from build123d import *

# Parameters (mm, degrees)
BOSS_EXTRUDE1_DEPTH        = 10
M4_TAPPED_HOLE1_AT_2_COUNT = 2
M4_TAPPED_HOLE1_AT_2_PITCH = 113
SKETCH7_R                  = 4
CUT_EXTRUDE1_DEPTH         = 10
CUT_EXTRUDE1_DEPTH_BACK    = 6.6


with BuildPart() as part:
    # Sketch1 → Boss-Extrude1 (new body)
    with BuildSketch(Plane(origin=(0, 0, 0), x_dir=(0, 0, -1), z_dir=(1, 0, 0))):
        with BuildLine():
            Line((-30, 53.366656257), (-30, 49.295030175))
            ThreePointArc((-30, 49.295030175), (-30.184412971, 48.574453483), (-30.692307692, 48.031055043))
            ThreePointArc((-30.692307692, 48.031055043), (-44.960469582, 35.036497755), (-54.07472853, 18.025641026))
            ThreePointArc((-54.07472853, 18.025641026), (-54.620689683, 17.283131383), (-55.497747702, 17))
            Line((-55.497747702, 17), (-61.001524227, 17))
            Line((-61.001524227, 17), (-61.001524227, 2))
            Line((-61.001524227, 2), (-51.961524227, 2))
            ThreePointArc((-51.961524227, 2), (0, 52), (51.961524227, 2))
            Line((51.961524227, 2), (60.998475773, 2))
            Line((60.998475773, 2), (60.998475773, 17))
            Line((60.998475773, 17), (55.497747702, 17))
            ThreePointArc((55.497747702, 17), (54.620689683, 17.283131383), (54.07472853, 18.025641026))
            ThreePointArc((54.07472853, 18.025641026), (44.960469582, 35.036497755), (30.692307692, 48.031055043))
            ThreePointArc((30.692307692, 48.031055043), (30.184412971, 48.574453483), (30, 49.295030175))
            Line((30, 49.295030175), (30, 53.366656257))
            ThreePointArc((30, 53.366656257), (29.786451973, 54.138045472), (29.20661157, 54.689796494))
            ThreePointArc((29.20661157, 54.689796494), (0, 62), (-29.20661157, 54.689796494))
            ThreePointArc((-29.20661157, 54.689796494), (-29.786451973, 54.138045472), (-30, 53.366656257))
        make_face()
    extrude(amount=BOSS_EXTRUDE1_DEPTH)

    # Sketch4 → M4 Tapped Hole1 (revolve, cut)
    with BuildSketch(Plane(origin=(5, 17, -56.498475773), x_dir=(0, 0, 1), z_dir=(1, 0, 0))):
        Polygon((0, 0), (0, 21.091420021), (1.65, 20.1), (1.65, 0), align=None)
    m4_tapped_hole1 = revolve(axis=Axis((5, 23.35, -56.498475773), (0, -1, 0)), mode=Mode.SUBTRACT)

    # M4 Tapped Hole1 at 2: M4 Tapped Hole1 ×2
    with Locations(*[(0, 0, i * M4_TAPPED_HOLE1_AT_2_PITCH) for i in range(1, M4_TAPPED_HOLE1_AT_2_COUNT)]):
        add(m4_tapped_hole1, mode=Mode.SUBTRACT)

    # Sketch7 → Cut-Extrude1 (cut, two sides)
    with BuildSketch(Plane(origin=(0, 17, 0), x_dir=(1, 0, 0), z_dir=(0, 1, 0))) as cut_extrude1_sk:
        with Locations((5, 56.498475773)):
            Circle(SKETCH7_R)
        with Locations((5, -56.501524227)):
            Circle(SKETCH7_R)
    extrude(amount=CUT_EXTRUDE1_DEPTH, mode=Mode.SUBTRACT)
    extrude(cut_extrude1_sk.sketch, amount=-CUT_EXTRUDE1_DEPTH_BACK, mode=Mode.SUBTRACT)


solid = part.part
Work out the finished part from the listing and answer in its coordinate system (mm). A direction names the side the tool comes from. Give positions to 0.01 mm unless a question says otherwise; leave off trailing zeros. Loops run counter-clockwise (first coordinate to the right, second up) from the corner with the lowest first, then second, coordinate; pieces in that order, holes last. Notation, with made-up numbers: (21, 4.5) - (72, 4.5) arc R20 ccw to (72, 28.5) - close; hole circle Ø5 at (-32, -19). An arc over 180 degrees is marked (long way). Answer in a Markdown table with one row per item. Add a question column.
Q1. Determine the mould class of faces 1 (the flat face through (5, 2, 59)), 2 (the flat face through (10, 52, 5)), 3 (the flat face through (0, 52, 5)), 4 (the cylindrical face through (4.927, 6.259, 54.853)) for opening direction X: released by +X, released by -X, zero draft, split by the parting line, or undercut.
Q2. A tool of negligible diameter and unlimited length cuts with its end or side. For faces 5 (the cylindrical face through (5, 62, 0)), 6 (the flat face through (5, 9, -60.998)), 7 (the flat face through (4.9, 17, 60.7)), 8 (the flat face through (7, 10.4, -57)), 9 (the flat face through (5, 51, -30)), from which of +Z, -Z, +X, -X, +Y, -Y can it reach the whole face along a straight path? Write none if from no direction.
Q3. Consider line 1 along Z through (x, y) = (6.75, 12); line 2 along Z through (x, y) = (5, 14.5); line 3 along Z through (x, y) = (2, 8.5). Determine where each line is inside the solid, lowest interval first.
Q4. Each of these flat-tipped pins is pushed along its axis until it touches: P1, Ø3.5, axis at x = 6.5, y = 51, coming from the +Z side; P2, Ø3.5, axis at x = 2.5, y = 52, coming from the -Z side; P3, Ø5, axis at x = 5, z = 56.5, coming from the +Y side; P4, Ø10, axis at y = 50, z = 2.5, coming from the +X side. Where does it stop, or does it pass through?
Q5. The part is cut by section D-D (y = 24.5). Determine the outline of the cut face in (x, z), and give its area (3 significant figures).
Q6. The part is cut by section B-B (y = 13). Determine the outline of the cut face in (x, z), and give its area (3 significant figures).
Q7. The part is cut by section C-C (y = 42.5). Determine the outline of the cut face in (x, z).
Q8. The part is cut by section A-A (x = 5). State how many separate pieces and enclosed holes the cut face has, and give its area (3 significant figures).
Solution:
| question | item | result |
|---|---|---|
| 1 | face 1 | zero draft |
| 1 | face 2 | released by +X |
| 1 | face 3 | released by -X |
| 1 | face 4 | undercut |
| 2 | face 5 | +X, -X, +Y |
| 2 | face 6 | -Z, +X, -X, +Y, -Y |
| 2 | face 7 | +Z, +X, -X, +Y |
| 2 | face 8 | +Y |
| 2 | face 9 | -Z, +X, -X, +Y |
| 3 | line 1 | z = -61 to -60.1, -52.9 to -50.6, 50.6 to 52.9, 60.1 to 61 |
| 3 | line 2 | z = -61 to -60.5, -52.5 to -49.94, 49.94 to 52.5, 60.5 to 61 |
| 3 | line 3 | z = -61 to -51.3, 51.3 to 61 |
| 4 | P1 | stops at z = 30 |
| 4 | P2 | stops at z = -30 |
| 4 | P3 | stops at y = 10.4 |
| 4 | P4 | stops at x = 10 |
| 5 | outline | (0, -51.47) - (10, -51.47) - (10, -45.87) - (0, -45.87) - close; (0, 45.87) - (10, 45.87) - (10, 51.47) - (0, 51.47) - close |
| 5 | area | 112 mm² |
| 6 | outline | (0, -61) - (10, -61) - (10, -50.35) - (0, -50.35) - close; (0, 50.35) - (10, 50.35) - (10, 61) - (0, 61) - close; hole circle Ø8 at (5, -56.5); hole circle Ø8 at (5, 56.5) |
| 6 | area | 112 mm² |
| 7 | outline | (0, -37.98) - (10, -37.98) - (10, -29.96) - (0, -29.96) - close; (0, 29.96) - (10, 29.96) - (10, 37.98) - (0, 37.98) - close |
| 8 | separate pieces | 3 |
| 8 | enclosed holes | 0 |
| 8 | area | 1,130 mm² |
